Source: CAD feature listing. Evaluate the final solid. Frame: model axes, mm. A direction names the side the tool comes from. Round coordinates to 2 decimals unless told otherwise and drop trailing zeros. Write each loop counter-clockwise with the first axis right and the second up, starting at its lowest first coordinate (ties: lowest second). Pieces come first, ordered by that corner, then holes. Notation, with made-up numbers: (76, 19) -> (89, 19) arc R12 cw to (89, 38) -> close; hole circle Ø7 at (54, 79). An arc over 180 degrees is marked (long way). Return JSON: item names as keys, results as strings. Group by question number.
from build123d import *

# Parameters (mm, degrees)
BASE_FLANGE1_DEPTH = 10
CUT_EXTRUDE1_REACH = 155.346
SKETCH7_R          = 2.5
CUT_EXTRUDE2_REACH = 155.346


# Sheet-metal steps are written as plain solids
with BuildPart() as part:
    # Sketch2 → Base-Flange1 (new body)
    with BuildSketch(Plane.XY):
        with BuildLine():
            Line((7.5, 49.434299833), (7.5, 144.62))
            Line((7.5, 144.62), (-7.5, 144.62))
            Line((-7.5, 144.62), (-7.5, 49.434299833))
            ThreePointArc((-7.5, 49.434299833), (0, -50), (7.5, 49.434299833))
        make_face()
    extrude(amount=-BASE_FLANGE1_DEPTH)

    # Sketch7 → Cut-Extrude1 (cut, up to next)
    with BuildSketch(Plane.XY, mode=Mode.PRIVATE) as cut_extrude1_sk1:
        with Locations((0, 134.62)):
            Circle(SKETCH7_R)
    cut_extrude1_tool1 = extrude(cut_extrude1_sk1.sketch, amount=-CUT_EXTRUDE1_REACH, mode=Mode.PRIVATE) & part.part
    # Sketch7 → Cut-Extrude1 (cut, up to next)
    with BuildSketch(Plane.XY, mode=Mode.PRIVATE) as cut_extrude1_sk2:
        Circle(SKETCH7_R)
    cut_extrude1_tool2 = extrude(cut_extrude1_sk2.sketch, amount=-CUT_EXTRUDE1_REACH, mode=Mode.PRIVATE) & part.part
    add(cut_extrude1_tool1.solids().sort_by_distance((0, 134.62, 0))[0], mode=Mode.SUBTRACT)
    add(cut_extrude1_tool2.solids().sort_by_distance((0, 0, 0))[0], mode=Mode.SUBTRACT)

    # Sketch8 → Cut-Extrude2 (cut, up to next)
    with BuildSketch(Plane.XY, mode=Mode.PRIVATE) as cut_extrude2_sk1:
        with BuildLine():
            Line((7.5, 49.434299833), (7.871687465, 42.043640294))
            Line((7.871687465, 42.043640294), (10.372740004, 41.497438686))
            Line((10.372740004, 41.497438686), (13.791710294, 48.060261414))
            ThreePointArc((13.791710294, 48.060261414), (10.66800015, 48.848682406), (7.5, 49.434299833))
        make_face()
    cut_extrude2_tool1 = extrude(cut_extrude2_sk1.sketch, amount=-CUT_EXTRUDE2_REACH, mode=Mode.PRIVATE) & part.part
    add(cut_extrude2_tool1.solids().sort_by_distance((10.002556, 45.80162, 0))[0], mode=Mode.SUBTRACT)


solid = part.part
Item 1: First-contact query: pin 1 Ø1.5 at (y, z) = (-6, -3) entering from -X; pin 2 Ø3 at (x, z) = (-33.5, -2) entering from -Y; pin 3 Ø3 at (y, z) = (77.5, -5) entering from -X. Flat tips, straight axial feed; report the tip coordinate or a pass-through.
Item 2: Pull-direction query (Y, two-part tool) for faces 1 (the flat face through (7.683, 45.791, -4.93)), 2 (the cylindrical face through (1.34, 136.73, -4.93)), 3 (the flat face through (-1, 5, -10)); classes: +Y half, -Y half, draft (parallel to the pull), parting line (faces both ways), or undercut.
Item 3: Cut plane D-D on y = 134.62. Output: boundary loops of the cut face in (x, z), and give its area (3 significant figures).
Item 4: Cut plane C-C on x = 0. Output: boundary loops of the cut face in (y, z), and give its area (3 significant figures).
Item 5: Material intervals for probe 1 along Y at (x, z) = (0, -5.25); probe 2 along Y at (x, z) = (-1.5, -4.5); probe 3 along X at (y, z) = (134.62, -6.5), sorted ascending.
Item 6: Cut plane A-A on z = -7. Output: boundary loops of the cut face in (x, y).
Item 7: Set-up query: faces 4 (the flat face through (12.058, 44.733, -4.93)), 5 (the cylindrical face through (-5.261, -49.722, -4.93)), 6 (the flat face through (7.5, 96, -5)), 7 (the flat face through (-7.5, 98, -5)), 8 (the flat face through (0, 144.62, -5)). Return all of +Z, -Z, +X, -X, +Y, -Y with unobstructed straight access to the full face (end or side cutting, diameter ignored); none if empty.
Item 8: Cut plane B-B on y = 0. Output: boundary loops of the cut face in (x, z).
Here are the results:
{
 "1": {"pin 1": "stops at x = -49.72", "pin 2": "stops at y = -38.42", "pin 3": "stops at x = -7.5"},
 "2": {"face 1": "+Y half", "face 2": "undercut", "face 3": "draft"},
 "3": {"outline": "(-7.5, -10) -> (-2.5, -10) -> (-2.5, 0) -> (-7.5, 0) -> close; (2.5, -10) -> (7.5, -10) -> (7.5, 0) -> (2.5, 0) -> close", "area": "100 mm^2"},
 "4": {"outline": "(-50, -10) -> (-2.5, -10) -> (-2.5, 0) -> (-50, 0) -> close; (2.5, -10) -> (132.12, -10) -> (132.12, 0) -> (2.5, 0) -> close; (137.12, -10) -> (144.62, -10) -> (144.62, 0) -> (137.12, 0) -> close", "area": "1,850 mm^2"},
 "5": {"probe 1": "y = -50 to -2.5, 2.5 to 132.12, 137.12 to 144.62", "probe 2": "y = -49.98 to -2, 2 to 132.62, 136.62 to 144.62", "probe 3": "x = -7.5 to -2.5, 2.5 to 7.5"},
 "6": {"outline": "(-7.5, 49.43) arc R50 ccw (long way) to (13.79, 48.06) -> (10.37, 41.5) -> (7.87, 42.04) -> (7.5, 49.43) -> (7.5, 144.62) -> (-7.5, 144.62) -> close; hole circle Ø5 at (0, 0); hole circle Ø5 at (0, 134.62)"},
 "7": {"face 4": "+Z, -Z, +Y", "face 5": "+Z, -Z", "face 6": "+Z, -Z, +X, +Y", "face 7": "+Z, -Z, -X, +Y", "face 8": "+Z, -Z, +X, -X, +Y"},
 "8": {"outline": "(-50, -10) -> (-2.5, -10) -> (-2.5, 0) -> (-50, 0) -> close; (2.5, -10) -> (50, -10) -> (50, 0) -> (2.5, 0) -> close"}
}
